from build123d import *

# Parameters (mm, degrees)
SKETCH_1_R          = 50
EXTRUDE_3_DEPTH     = 45
SKETCH_5_R          = 5
CUT_EXTRUDE_1_DEPTH = 84.815273071
CUT_EXTRUDE_START   = -5
SKETCH_6_R          = 50
CUT_EXTRUDE_2_DEPTH = 5
SCALE_3_SCALE       = 0.5
SCALE_4_SCALE       = 1.2
SKETCH_7_R          = 30
SKETCH_7_R_2        = 3
EXTRUDE_4_DEPTH     = 2.4


with BuildPart() as part:
    # 草图1 → 凸台-拉伸3 (new body)
    with BuildSketch(Plane(origin=(0, 0, 0), x_dir=(1, 0, 0), z_dir=(0, 1, 0))):
        with Locations(Location((0, 0, 0), (0, 0, 90))):
            Circle(SKETCH_1_R)
    extrude(amount=EXTRUDE_3_DEPTH)

    # 草图5 → 切除-拉伸1 (cut, through all)
    with BuildSketch(Plane.XZ):
        with Locations(Location((0, 0, 0), (0, 0, 270))):
            Circle(SKETCH_5_R)
    extrude(amount=-CUT_EXTRUDE_1_DEPTH, mode=Mode.SUBTRACT)

    # 草图6 → 切除-拉伸2 (cut)
    with BuildSketch(Plane(origin=(0, 45, 0), x_dir=(1, 0, 0), z_dir=(0, 1, 0)).offset(CUT_EXTRUDE_START)):
        with Locations(Location((0, 0, 0), (0, 0, 90))):
            Circle(SKETCH_6_R)
    extrude(amount=CUT_EXTRUDE_2_DEPTH, mode=Mode.SUBTRACT)


with BuildPart() as part_1:
    # 缩放比例3: scaled about (0, 20, 0)
    add(part.part.scale(SCALE_3_SCALE).moved(Location((0, 10, 0))))


with BuildPart() as part_2:
    # 缩放比例4: scaled about (0, 20, 0)
    add(part_1.part.scale(SCALE_4_SCALE).moved(Location((0, -4, 0))))

    # 草图7 → 凸台-拉伸4 (add)
    with BuildSketch(Plane(origin=(0, 32, 0), x_dir=(1, 0, 0), z_dir=(0, 1, 0))):
        with Locations(Location((0, 0, 0), (0, 0, 90))):
            Circle(SKETCH_7_R)
        with Locations(Location((0, 0, 0), (0, 0, 90))):
            Circle(SKETCH_7_R_2, mode=Mode.SUBTRACT)
    extrude(amount=EXTRUDE_4_DEPTH)


solid = part_2.part
Read the model definition and answer for the solid it produces. Units are mm, in the model's axes. Round coordinates to 2 decimals unless told otherwise and drop trailing zeros. Order: outer loops, then holes, each group sorted by start corner. A loop starts at its lowest first (then second) coordinate and runs counter-clockwise, first axis right, second up.
1) The part is cut by section D-D on z = 18. Write down the section's boundary in (x, y), plus the area to 3 significant figures.
2) The mould has two halves that part along X. Classify faces 1 (the face through (0, 8, -6)), 2 (the face through (-0.9, 21.02, -2.86)), 3 (the face through (-1.32, 21.02, 29.97)): released by +X, released by -X, zero draft, split by the parting line, or undercut.
3) The part is cut by section C-C on y = 10.25. Write down the section's boundary in (x, z), plus the area to 3 significant figures.
4) Straight lines are drawn through the part: L1, parallel to X at y = 17.5, z = 0; L2, parallel to Z at x = 2, y = 33.5; L3, parallel to X at y = 26, z = 27.5. For each, find the intervals that lie inside material, in ascending order.
5) The part is cut by section B-B on x = 0. Write down the section's boundary in (y, z).
6) The part is cut by section A-A on z = 0. Write down the section's boundary in (x, y), plus the area to 3 significant figures.
7) Flat-ended cylindrical pins translate along their axes: pin 1 (1 mm diameter, centred on x = 8.5, y = 27.5, fed in from +Z); pin 2 (2 mm diameter, centred on x = 15, y = 23.5, fed in from -Z); pin 3 (3 mm diameter, centred on y = 17, z = -14, fed in from -X). Find the tip coordinate at first contact, or state that the pin passes through.
Resolved:
1. outline: (-24, 8) - (24, 8) - (24, 34.4) - (-24, 34.4) - close
1. area: 1,270 mm2
2. face 1: zero draft
2. face 2: undercut
2. face 3: split by the parting line
3. outline: circle Ø60 at (0, 0); hole circle Ø6 at (0, 0)
3. area: 2,800 mm2
4. L1: x = -30 to -3, 3 to 30
4. L2: z = -29.93 to -2.24, 2.24 to 29.93
4. L3: x = -11.99 to 11.99
5. outline: (8, -30) - (34.4, -30) - (34.4, -3) - (8, -3) - close; (8, 3) - (34.4, 3) - (34.4, 30) - (8, 30) - close
6. outline: (-30, 8) - (-3, 8) - (-3, 34.4) - (-30, 34.4) - close; (3, 8) - (30, 8) - (30, 34.4) - (3, 34.4) - close
6. area: 1,430 mm2
7. pin 1: stops at z = 28.91
7. pin 2: stops at z = -26.53
7. pin 3: stops at x = -27.27
